from build123d import *

# Parameters (mm, degrees)
F1_DEPTH = 8


# Not quite as in the source:
# - ends of sketch curves that miss each other by under 0.0002 mm in the source are joined


with BuildPart() as f1:
    # F0 (on Front) → F1 (new body)
    with BuildSketch(Plane.XZ):
        with BuildLine():
            Line((76, -164), (76, -239.943211))
            Line((76, -239.943211), (72.5, -242.910554))
            Line((72.5, -242.910554), (72.5, -329))
            ThreePointArc((72.5, -329), (124.1533829832, -321.067337789), (175.0000000351, -309.0000001251))
            Line((175.0000000351, -309.0000001251), (169.278269, -284.66357))
            Line((169.278269, -284.66357), (110.870838, -298.395725))
            ThreePointArc((110.870838, -298.395725), (86.8243094388, -283.5039655144), (101.716068848, -259.4574373536))
            Line((101.716068848, -259.4574373536), (160.123499, -245.725283))
            Line((160.123499, -245.725283), (100, 10))
            Line((100, 10), (129.421287, 41.816044))
            Line((129.421287, 41.816044), (85.369419, 82.552181))
            ThreePointArc((85.369419, 82.552181), (84.2641744646, 110.8148490327), (112.5268427835, 111.9200937658))
            Line((112.5268427835, 111.9200937658), (156.578712, 71.183957))
            Line((156.578712, 71.183957), (186, 103))
            Line((186, 103), (189.810038, 142.094309))
            Line((189.810038, 142.094309), (130.092964, 147.914193))
            ThreePointArc((130.092964, 147.914193), (112.1272346173, 169.7598464886), (133.9728870415, 187.7255764263))
            Line((133.9728870415, 187.7255764263), (193.689961, 181.905692))
            Line((193.689961, 181.905692), (197.5, 221))
            Line((197.5, 221), (169.928822, 250.409256))
            Line((169.928822, 250.409256), (126.15659, 209.372789))
            ThreePointArc((126.15659, 209.372789), (97.8870239172, 210.2847104224), (98.7989451563, 238.5542768333))
            Line((98.7989451563, 238.5542768333), (142.571177, 279.590745))
            Line((142.571177, 279.590745), (115, 309))
            Line((115, 309), (77.204235, 315.573177))
            Line((77.204235, 315.573177), (66.923764, 256.460472))
            ThreePointArc((66.923764, 256.460472), (43.7927054839, 240.1830599073), (27.5152939917, 263.3141190014))
            Line((27.5152939917, 263.3141190014), (37.795765, 322.426824))
            Line((37.795765, 322.426824), (0, 329))
            Line((0, 329), (-37.795765, 322.426824))
            Line((-37.795765, 322.426824), (-27.515295, 263.314119))
            ThreePointArc((-27.515295, 263.314119), (-43.7927064839, 240.1830599073), (-66.9237651771, 256.4604719692))
            Line((-66.9237651771, 256.4604719692), (-77.204235, 315.573177))
            Line((-77.204235, 315.573177), (-115, 309))
            Line((-115, 309), (-142.571178, 279.590745))
            Line((-142.571178, 279.590745), (-98.798945, 238.554277))
            ThreePointArc((-98.798945, 238.554277), (-97.8870241667, 210.2847101563), (-126.1565908437, 209.3727891667))
            Line((-126.1565908437, 209.3727891667), (-169.928823, 250.409256))
            Line((-169.928823, 250.409256), (-197.5, 221))
            Line((-197.5, 221), (-193.689962, 181.905692))
            Line((-193.689962, 181.905692), (-133.972888, 187.725576))
            ThreePointArc((-133.972888, 187.725576), (-112.1272346173, 169.7598464886), (-130.092965055, 147.9141935643))
            Line((-130.092965055, 147.9141935643), (-189.810039, 142.094309))
            Line((-189.810039, 142.094309), (-186, 103))
            Line((-186, 103), (-156.578713, 71.183957))
            Line((-156.578713, 71.183957), (-112.526844, 111.920094))
            ThreePointArc((-112.526844, 111.920094), (-84.2641747139, 110.8148493022), (-85.3694187181, 82.5521806951))
            Line((-85.3694187181, 82.5521806951), (-129.421288, 41.816044))
            Line((-129.421288, 41.816044), (-100, 10))
            Line((-100, 10), (-160.1235, -245.725283))
            Line((-160.1235, -245.725283), (-101.716069, -259.457438))
            ThreePointArc((-101.716069, -259.457438), (-86.8243105502, -283.5039659882), (-110.8708388768, -298.395724476))
            Line((-110.8708388768, -298.395724476), (-169.278269, -284.66357))
            Line((-169.278269, -284.66357), (-175, -309))
            ThreePointArc((-175, -309), (-124.1533829832, -321.067337789), (-72.5000000145, -329.0000001291))
            Line((-72.5000000145, -329.0000001291), (-72.5, -242.910554))
            Line((-72.5, -242.910554), (-76, -239.943211))
            Line((-76, -239.943211), (-76, -164))
            ThreePointArc((-76, -164), (-73.0710678119, -156.9289321881), (-66, -154))
            Line((-66, -154), (0, -154))
            Line((0, -154), (66, -154))
            ThreePointArc((66, -154), (73.0710678119, -156.9289321881), (76, -164))
        make_face()
        with BuildLine():
            Line((65.800007, -18.166468), (0, -18.166468))
            Line((0, -18.166468), (-65.800008, -18.166468))
            ThreePointArc((-65.800008, -18.166468), (-72.3053903869, -15.4718503869), (-75.000008, -8.966468))
            Line((-75.000008, -8.966468), (-75.000008, 57.633575))
            ThreePointArc((-75.000008, 57.633575), (-72.3053903869, 64.1389573869), (-65.800008, 66.833575))
            Line((-65.800008, 66.833575), (0, 66.833575))
            Line((0, 66.833575), (65.800007, 66.833575))
            ThreePointArc((65.800007, 66.833575), (72.3053893869, 64.1389573869), (75.000007, 57.633575))
            Line((75.000007, 57.633575), (75.000007, -8.966468))
            ThreePointArc((75.000007, -8.966468), (72.3053893869, -15.4718503869), (65.800007, -18.166468))
        make_face(mode=Mode.SUBTRACT)
    extrude(amount=F1_DEPTH)

    # F3: sweep along a path in F3_path
    with BuildLine(Plane(origin=(110.870838, -8, -298.395725), x_dir=(0, 0, 1), z_dir=(0, -1, 0))) as f3_path:
        Line((13.732155, -58.407431), (0, 0))
        ThreePointArc((0, 0), (14.8917592236, 24.0465284996), (38.9382876464, 9.154769152))
        Line((38.9382876464, 9.154769152), (52.670442, -49.252661))
    # F2 (on face) → F3 (sweep, cut)
    with BuildSketch(Plane(origin=(96.989833717, 0, 22.8032516792), x_dir=(0, 1, 0), z_dir=(0.973457176, 0, 0.2288692344))):
        Polygon((0, -315.8503827909), (-8, -315.8503827909), (-8, -323.8503827909), align=None)
    sweep(path=f3_path.line, mode=Mode.SUBTRACT)

    # F5: sweep along a path in F5_path
    with BuildLine(Plane(origin=(85.369419, -8, 82.552181), x_dir=(0, 0, 1), z_dir=(0, -1, 0))) as f5_path:
        Line((-40.736137, -44.051868), (0, 0))
        ThreePointArc((0, 0), (28.2626681852, 1.1052443944), (29.3679127658, -27.1574237835))
        Line((29.3679127658, -27.1574237835), (-11.368224, -71.209293))
    # F4 (on face) → F5 (sweep, cut)
    with BuildSketch(Plane(origin=(48.9199144477, 0, -45.2377688119), x_dir=(0, 1, 0), z_dir=(0.7341978267, 0, -0.6789356017))):
        Polygon((0, 118.5699679847), (-8, 118.5699679847), (-8, 110.5699679847), align=None)
    sweep(path=f5_path.line, mode=Mode.SUBTRACT)

    # F7: sweep along a path in F7_path
    with BuildLine(Plane(origin=(130.092964, -8, 147.914193), x_dir=(0, 0, 1), z_dir=(0, -1, 0))) as f7_path:
        Line((-5.819884, -59.717074), (0, 0))
        ThreePointArc((0, 0), (21.8456531581, 17.9657294149), (39.8113834263, -3.8799230415))
        Line((39.8113834263, -3.8799230415), (33.991499, -63.596997))
    # F6 (on face) → F7 (sweep, cut)
    with BuildSketch(Plane(origin=(174.3063070687, 0, -16.9874764527), x_dir=(0, 1, 0), z_dir=(0.9952845708, 0, -0.0969980576))):
        Polygon((0, 159.8354783382), (-8, 159.8354783382), (-8, 151.8354783382), align=None)
    sweep(path=f7_path.line, mode=Mode.SUBTRACT)

    # F9: sweep along a path in F9_path
    with BuildLine(Plane(origin=(126.15659, -8, 209.372789), x_dir=(0, 0, 1), z_dir=(0, -1, 0))) as f9_path:
        Line((41.036467, -43.772232), (0, 0))
        ThreePointArc((0, 0), (0.9119215885, 28.2695662386), (29.1814878333, 27.3576448437))
        Line((29.1814878333, 27.3576448437), (70.217956, -16.414587))
    # F8 (on face) → F9 (sweep, cut)
    with BuildSketch(Plane(origin=(215.3846137301, 0, 201.9230790338), x_dir=(0, 1, 0), z_dir=(0.729537198, 0, 0.6839411355))):
        Polygon((0, 66.4615554934), (-8, 66.4615554934), (-8, 58.4615554934), align=None)
    sweep(path=f9_path.line, mode=Mode.SUBTRACT)

    # F11: sweep along a path in F11_path
    with BuildLine(Plane(origin=(66.923764, -8, 256.460472), x_dir=(0, 0, 1), z_dir=(0, -1, 0))) as f11_path:
        Line((59.112705, -10.280471), (0, 0))
        ThreePointArc((0, 0), (-16.2774120773, 23.1310586047), (6.8536470014, 39.4084700083))
        Line((6.8536470014, 39.4084700083), (65.966352, 29.127999))
    # F10 (on face) → F11 (sweep, cut)
    with BuildSketch(Plane(origin=(55.5376187282, 0, 319.3412844519), x_dir=(0.9852117527, 0, -0.1713411869), z_dir=(0.1713411869, 0, 0.9852117527))):
        Polygon((21.9918369956, 0), (21.9918369956, -8), (29.9918369956, -8), align=None)
    sweep(path=f11_path.line, mode=Mode.SUBTRACT)

    # F13: sweep along a path in F13_path
    with BuildLine(Plane(origin=(-27.515295, -8, 263.314119), x_dir=(0, 0, 1), z_dir=(0, -1, 0))) as f13_path:
        Line((59.112705, 10.28047), (0, 0))
        ThreePointArc((0, 0), (-23.1310590934, 16.277411488), (-6.8536470308, 39.4084701771))
        Line((-6.8536470308, 39.4084701771), (52.259058, 49.68894))
    # F12 (on face) → F13 (sweep, cut)
    with BuildSketch(Plane(origin=(-55.5376105295, 0, 319.341285892), x_dir=(0.9852117571, 0, 0.1713411616), z_dir=(-0.1713411616, 0, 0.9852117571))):
        Polygon((18.008154492, 0), (18.008154492, -8), (26.008154492, -8), align=None)
    sweep(path=f13_path.line, mode=Mode.SUBTRACT)

    # F15: sweep along a path in F15_path
    with BuildLine(Plane(origin=(-126.1565908437, -8, 209.3727891667), x_dir=(0, 0, -1), z_dir=(0, 1, 0))) as f15_path:
        Line((-41.0364668333, 43.7722321563), (0, 0))
        ThreePointArc((0, 0), (-0.9119210729, -28.2695667552), (-29.1814878333, -27.3576458437))
        Line((-29.1814878333, -27.3576458437), (-70.2179558333, 16.4145871563))
    # F14 (on face) → F15 (sweep, cut)
    with BuildSketch(Plane(origin=(-215.3846129172, 0, 201.9230851377), x_dir=(0, -1, 0), z_dir=(-0.7295371863, 0, 0.6839411479))):
        Polygon((0, 106.461550303), (8, 106.461550303), (8, 114.461550303), align=None)
    sweep(path=f15_path.line, mode=Mode.SUBTRACT)

    # F17: sweep along a path in F17_path
    with BuildLine(Plane(origin=(-133.972888, -8, 187.725576), x_dir=(0, 0, 1), z_dir=(0, -1, 0))) as f17_path:
        Line((-5.819884, 59.717074), (0, 0))
        ThreePointArc((0, 0), (-17.9657296763, -21.8456533988), (-39.8113824357, -3.879922945))
        Line((-39.8113824357, -3.879922945), (-45.631267, 55.837151))
    # F16 (on face) → F17 (sweep, cut)
    with BuildSketch(Plane(origin=(-174.3063082, 0, -16.9874769975), x_dir=(0, -1, 0), z_dir=(-0.9952845705, 0, -0.09699806))):
        Polygon((0, 199.8354791034), (8, 199.8354791034), (8, 207.8354791034), align=None)
    sweep(path=f17_path.line, mode=Mode.SUBTRACT)

    # F19: sweep along a path in F19_path
    with BuildLine(Plane(origin=(-112.526844, -8, 111.920094), x_dir=(0, 0, 1), z_dir=(0, -1, 0))) as f19_path:
        Line((-40.736137, 44.051869), (0, 0))
        ThreePointArc((0, 0), (-1.1052443315, -28.2626689474), (-29.3679133049, -27.1574252819))
        Line((-29.3679133049, -27.1574252819), (-70.10405, 16.894444))
    # F18 (on face) → F19 (sweep, cut)
    with BuildSketch(Plane(origin=(-48.9199129921, 0, -45.2377688877), x_dir=(0, -1, 0), z_dir=(-0.7341978161, 0, -0.6789356132))):
        Polygon((0, 158.5699702901), (8, 158.5699702901), (8, 166.5699702901), align=None)
    sweep(path=f19_path.line, mode=Mode.SUBTRACT)

    # F21: sweep along a path in F21_path
    with BuildLine(Plane(origin=(-101.716069, -8, -259.457438), x_dir=(0, 0, 1), z_dir=(0, -1, 0))) as f21_path:
        Line((13.732155, 58.407431), (0, 0))
        ThreePointArc((0, 0), (-24.0465282, -14.8917584), (-38.938286476, 9.1547698768))
        Line((-38.938286476, 9.1547698768), (-25.206132, 67.5622))
    # F20 (on face) → F21 (sweep, cut)
    with BuildSketch(Plane(origin=(-96.9898309629, 0, 22.8032521208), x_dir=(0, -1, 0), z_dir=(-0.9734571736, 0, 0.2288692447))):
        Polygon((0, -275.8503839769), (8, -275.8503839769), (8, -267.8503839769), align=None)
    sweep(path=f21_path.line, mode=Mode.SUBTRACT)


solid = f1.part
Could you check a few things on this model? Use its own coordinates, in mm. A direction names the side the tool comes from. Give positions to 0.01 mm unless a question says otherwise; leave off trailing zeros. Order: outer loops, then holes, each group sorted by start corner. A loop starts at its lowest first (then second) coordinate and runs counter-clockwise, first axis right, second up.
Item 1: If we mould it in two halves opening along Z, with no side actions, what happens to faces 1 (the face through (-124.872, -3.944, -320.927)), 2 (the face through (164.643, -4.056, 188.812)), 3 (the face through (-183.52, -3.94, 235.91)), 4 (the face through (28.73, -4.06, 293.98))? For each: pulls with the +Z half, pulls with the -Z half, needs draft (parallel to the pull), parting line crosses it, or undercut.
Item 2: For faces 5 (the face through (114.505, -3.944, 25.685)), 6 (the face through (-171.495, -3.944, 87.315)), 7 (the face through (-163.807, -4.056, 188.893)), 8 (the face through (-159.976, -4.056, 140.927)), 9 (the face through (-3, 0, 78)), which set-ups out of +Z, -Z, +X, -X, +Y, -Y let a thin tool reach every point of the face, with its end or its side?
Item 3: I'm going to push flat-ended pins straight in: pin 1 (3 mm diameter, centred on x = -52.5, y = -6, fed in from +Z); pin 2 (1 mm diameter, centred on y = -4.5, z = -190, fed in from +X); pin 3 (1.5 mm diameter, centred on x = 133, y = -6.5, fed in from +Z). Where does each tip first touch, or does it pass through?
Item 4: I need wall thicknesses on line 1 (X direction, y = -7.5, z = 263); line 2 (X direction, y = -2.25, z = 241); line 3 (Z direction, x = 159.5, y = -7.25). Which ranges of each line are inside material? Lowest first, please.
Item 5: If we section it at A-A, the plane z = -109: Write out the boundary of the cut face in (x, y).
Item 6: If we section it at B-B, the plane z = 90: Count the separate pieces of the cut face and the enclosed holes in it, plus the area to 3 significant figures.
Values:
1. face 1: pulls with the -Z half
1. face 2: undercut
1. face 3: pulls with the +Z half
1. face 4: undercut
2. face 5: +X, +Y, -Y
2. face 6: -X, +Y, -Y
2. face 7: -Y
2. face 8: -X, -Y
2. face 9: +Z, -Z, +X, -X, +Y
3. pin 1: stops at z = 236
3. pin 2: stops at x = 147.14
3. pin 3: stops at z = 290.6
4. line 1: x = -113.91 to -75.67, -19.9 to 19.9, 75.67 to 113.91
4. line 2: x = -178.75 to -163.18, -98.12 to -58.98, -35.46 to 35.46, 58.98 to 98.12, 163.18 to 178.75
4. line 3: z = -313.14 to -294.41, 78.36 to 137.76, 192.52 to 230.69
5. outline: (-127.98, -8) - (127.98, -8) - (127.98, 0) - (-127.98, 0) - close
6. separate pieces: 3
6. enclosed holes: 0
6. area: 1,730 mm2
